```python
from build123d import *

# Parameters (mm, degrees)
F0_R      = 25.4
F1_DEPTH  = 22.225
F2_R      = 31.75
F3_DEPTH  = 6.35
F4_W      = 68.9518330619
F4_H      = 1.524
F5_DEPTH  = 44.451
F7_R      = 5.55625
F8_DEPTH  = 50.8
F10_D     = 7.14375
F12_D     = 5.1054
F12_DEPTH = 19.05
F12_TIP   = 1.5338169022


with BuildPart() as f1:
    # F0 (on Right) → F1 (new body, symmetric)
    with BuildSketch(Plane.YZ):
        with BuildLine():
            Line((35.9210244843, 44.45), (-35.9210244843, 44.45))
            ThreePointArc((-35.9210244843, 44.45), (-57.15, 0), (-35.9210244843, -44.45))
            Line((-35.9210244843, -44.45), (35.9210244843, -44.45))
            ThreePointArc((35.9210244843, -44.45), (57.15, 0), (35.9210244843, 44.45))
        make_face()
        Circle(F0_R, mode=Mode.SUBTRACT)
    extrude(amount=F1_DEPTH, both=True)

    # F2 (on face) → F3 (cut)
    with BuildSketch(Plane.YZ.offset(22.225)):
        Circle(F2_R)
    extrude(amount=-F3_DEPTH, mode=Mode.SUBTRACT)

    # F4 (on face) → F5 (cut, through all)
    with BuildSketch(Plane.YZ.offset(22.225)):
        with Locations((39.5418689586, 0.762)):
            Rectangle(F4_W, F4_H)
        with Locations((39.5418689586, -0.762)):
            Rectangle(F4_W, F4_H)
    extrude(amount=-F5_DEPTH, mode=Mode.SUBTRACT)

    # F7 (on offset) → F8 (cut)
    with BuildSketch(Plane.XY.offset(9.652)):
        with Locations((12.7, 44.4296763863)):
            Circle(F7_R)
        with Locations((-12.7, 44.4296763863)):
            Circle(F7_R)
    extrude(amount=F8_DEPTH, mode=Mode.SUBTRACT)

    # F10 (through all)
    with Locations(Plane.XY.offset(9.652)):
        with Locations((-12.7, 44.4296763863), (12.7, 44.4296763863)):
            Hole(F10_D / 2)

    # F12
    with Locations(Plane.YZ.offset(22.225)):
        with Locations((0, 38.1), (32.9955678842, -19.05), (-32.9955678842, -19.05)):
            Hole(F12_D / 2, depth=F12_DEPTH)
            with Locations((0, 0, -(F12_DEPTH + F12_TIP / 2))):  # 118° drill point
                Cone(0, F12_D / 2, F12_TIP, mode=Mode.SUBTRACT)


solid = f1.part
```
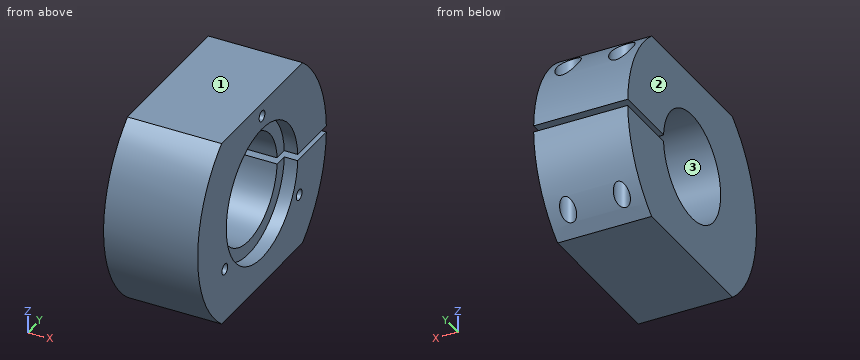
Source: CAD feature listing. Evaluate the final solid. Frame: model axes, mm. Face numbers are marked on the shaded views. Round coordinates to 2 decimals unless told otherwise and drop trailing zeros. Loops run counter-clockwise (first coordinate to the right, second up) from the corner with the lowest first, then second, coordinate; pieces in that order, holes last.
(1) Section query B-B (x = 12.7). Output: boundary loops of the cut face in (y, z).
From the geometry:
outline: (-35.92, -44.45) - (35.92, -44.45) arc R57.15 ccw to (40.86, -39.96) - (40.86, -1.52) - (25.35, -1.52) arc R25.4 cw (long way) to (25.35, 1.52) - (40.86, 1.52) - (40.86, 9.65) - (38.87, 9.65) - (38.87, 41.89) arc R57.15 ccw to (35.92, 44.45) - (-35.92, 44.45) arc R57.15 ccw to start; (48, -31.02) arc R57.15 ccw to (57.13, -1.52) - (48, -1.52) - close; (48, 1.52) - (57.13, 1.52) arc R57.15 ccw to (49.99, 27.7) - (49.99, 9.65) - (48, 9.65) - close; hole circle Ø5.11 at (-33, -19.05); hole circle Ø5.11 at (0, 38.1); hole circle Ø5.11 at (33, -19.05)
(2) Section query C-C (x = -2.5). Output: boundary loops of the cut face in (y, z).
From the geometry:
outline: (-35.92, -44.45) - (35.92, -44.45) arc R57.15 ccw to (57.13, -1.52) - (25.35, -1.52) arc R25.4 cw (long way) to (25.35, 1.52) - (57.13, 1.52) arc R57.15 ccw to (35.92, 44.45) - (-35.92, 44.45) arc R57.15 ccw to start
(3) Pull-direction query (Z, two-part tool) for the marked faces 1, 2 and 3; classes: +Z half, -Z half, draft (parallel to the pull), parting line (faces both ways), or undercut.
From the geometry:
face 1: +Z half
face 2: draft
face 3: undercut
(4) Material intervals for probe 1 along Y at (x, z) = (13.5, 8.5); probe 2 along Y at (x, z) = (11, -19); probe 3 along Y at (x, z) = (15, -13), sorted ascending.
From the geometry:
probe 1: y = -56.51 to -23.94, 23.94 to 40.95, 47.91 to 56.51
probe 2: y = -53.9 to -35.55, -30.44 to -16.86, 16.86 to 30.44, 35.55 to 41.29, 47.57 to 53.9
probe 3: y = -55.65 to -21.82, 21.82 to 41.7, 47.16 to 55.65
(5) Section query D-D (y = 18). Output: boundary loops of the cut face in (x, z) (3 decimals).
From the geometry:
outline: (-22.225, -44.45) - (22.225, -44.45) - (22.225, -26.155) - (15.875, -26.155) - (15.875, -17.921) - (-22.225, -17.921) - close; (-22.225, 17.921) - (15.875, 17.921) - (15.875, 26.155) - (22.225, 26.155) - (22.225, 44.45) - (-22.225, 44.45) - close
(6) Section query A-A (z = -23). Output: boundary loops of the cut face in (x, y) (1 decimal), and give its area (3 significant figures).
From the geometry:
outline: (-22.2, -52.3) - (22.2, -52.3) - (22.2, -21.9) - (15.9, -21.9) - (15.9, -10.8) - (-22.2, -10.8) - close; (-22.2, 10.8) - (15.9, 10.8) - (15.9, 21.9) - (22.2, 21.9) - (22.2, 52.3) - (-22.2, 52.3) - close; hole circle Ø7.1 at (-12.7, 44.4); hole circle Ø7.1 at (12.7, 44.4)
area: 3,470 mm2
(7) Contact query for flat-ended pins moving along their axis: pin 1 Ø3 at (x, y) = (6, 41.5) entering from +Z; pin 2 Ø5.5 at (x, y) = (-12.7, 44.43) entering from -Z; pin 3 Ø12 at (x, z) = (1.5, 30.5) entering from +Y; pin 4 Ø11.5 at (x, y) = (-12.7, 44.43) entering from -Z. Output: stop coordinate, or through.
From the geometry:
pin 1: stops at z = 40.82
pin 2: passes through
pin 3: stops at y = 51.63
pin 4: stops at z = -42.07
